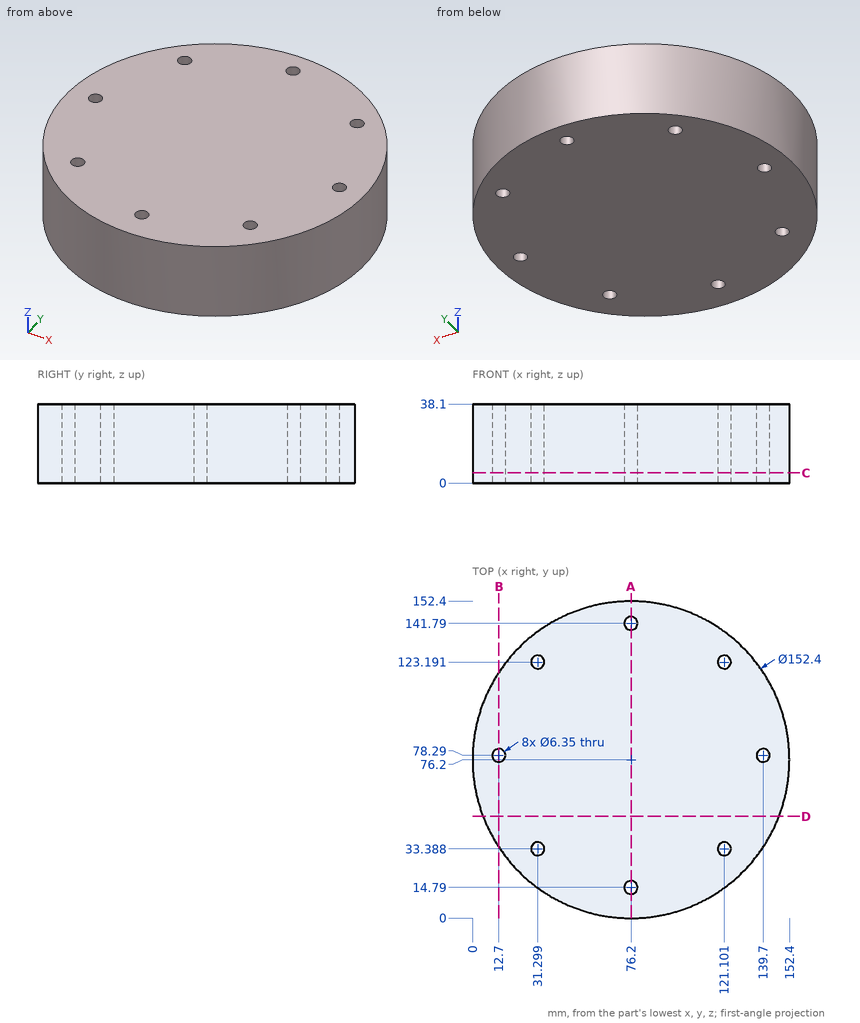
Geometry check sheet. Reference: drawing and pictorial views, mm from the part's lowest x, y, z. Give positions to 0.01 mm unless a question says otherwise; leave off trailing zeros. Write each loop counter-clockwise with the first axis right and the second up, starting at its lowest first coordinate (ties: lowest second). Pieces come first, ordered by that corner, then holes.
Item 1: Scan lines: L1, parallel to Y at x = 30, z = 10.5 (1 decimal); L2, parallel to Y at x = 74, z = 17; L3, parallel to X at y = 139.5, z = 5. Record each from-to range of solid material in increasing order.
Item 2: Cross-section at D-D (y = 49). Enter the section's corners in (x, z), and give its area (3 significant figures).
Item 3: Cross-section at B-B (x = 12.7). Enter the section's corners in (y, z) (1 decimal), and give its area (3 significant figures).
Item 4: Cross-section at A-A (x = 76.2). Enter the section's corners in (y, z) (1 decimal).
Item 5: Cross-section at C-C (z = 5). Count the separate pieces of the cut face and the enclosed holes in it, and give its area (3 significant figures).
Item 6: Gauge pin test, flat ends, axial feed: pin 1 (10 mm diameter, centred on x = 26.5, z = 19, fed in from +Y); pin 2 (8 mm diameter, centred on x = 28.5, z = 34, fed in from +Y) (1 decimal); pin 3 (5 mm diameter, centred on x = 68, z = 21.5, fed in from +Y). Record the tip position at first contact, or that the pin passes through.
Report:
1. L1: y = 15.6 to 30.5, 36.3 to 120.3, 126.1 to 136.8
1. L2: y = 0.03 to 12.5, 17.08 to 139.5, 144.08 to 152.37
1. L3: x = 33.78 to 74, 78.4 to 118.62
2. outline: (5.02, 0) - (147.38, 0) - (147.38, 38.1) - (5.02, 38.1) - close
2. area: 5,420 mm2
3. outline: (34.1, 0) - (75.1, 0) - (75.1, 38.1) - (34.1, 38.1) - close; (81.5, 0) - (118.3, 0) - (118.3, 38.1) - (81.5, 38.1) - close
3. area: 2,970 mm2
4. outline: (0, 0) - (11.6, 0) - (11.6, 38.1) - (0, 38.1) - close; (18, 0) - (138.6, 0) - (138.6, 38.1) - (18, 38.1) - close; (145, 0) - (152.4, 0) - (152.4, 38.1) - (145, 38.1) - close
5. separate pieces: 1
5. enclosed holes: 8
5. area: 18,000 mm2
6. pin 1: stops at y = 137.91
6. pin 2: stops at y = 138.6
6. pin 3: stops at y = 152.19
